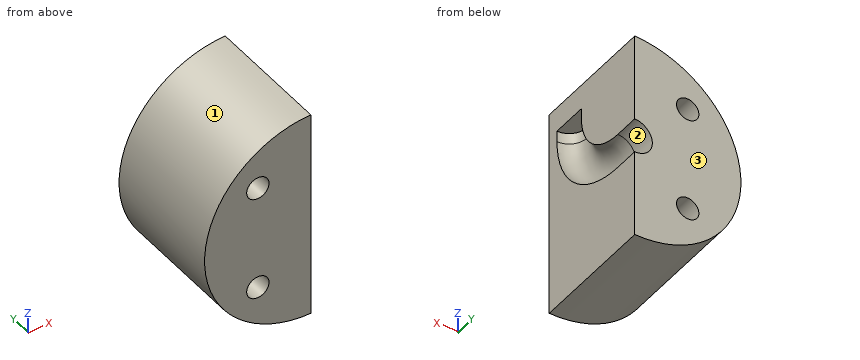
Autodesk Inventor part; units mm, degrees
ref_plane "YZ Plane" through (0, 0, 0) normal (1, 0, 0) x (0, 1, 0)
ref_plane "XZ Plane" through (0, 0, 0) normal (0, 1, 0) x (-1, 0, 0)
ref_plane "XY Plane" through (0, 0, 0) normal (0, 0, 1) x (1, 0, 0)
sketch "Sketch1" plane through (0, 0, 0) normal (0, 1, 0) x (-1, 0, 0)
  circle A0 centre (0, 0) radius 12.065
  line L0 (0, 0) -> (6.0168, -6.0168)
  line L1 (0, 0) -> (8.509, 0) construction
  circle A1 centre (6.0168, -6.0168) radius 1.27
  circle A2 centre (6.0168, 6.0168) radius 1.27
  circle A3 centre (-6.0168, 6.0168) radius 1.27
  circle A4 centre (-6.0168, -6.0168) radius 1.27
  dimension "d0" = 24.13
  dimension "d1" = 45
  dimension "d2" = 8.509
  dimension "d3" = 2.54
  dimension "d6" = 360
extrude "Extrusion1" add sketch "Sketch1" along normal blind 13.97
sketch "Sketch2" plane through (0, 0, 0) normal (1, 0, 0) x (0, 1, 0)
  line L0 (13.97, -12.065) -> (13.97, 12.065)
  line L1 (13.97, 0) -> (11.2075, 0)
  line L2 (11.2075, 0) -> (3.27, 0)
  line L3 (3.27, 0) -> (3.27, 7.9375)
  line L4 (3.27, 7.9375) -> (3.27, 9.2075)
  line L5 (0, 12.065) -> (0, -12.065)
  arc A0 (3.27, 7.9375) -> (11.2075, 0) centre (11.2075, 7.9375) ccw
  point P0 (0, 0)
  dimension "d15" = 7.9375
  dimension "d16" = 7.9375
  dimension "d17" = 1.27
  dimension "d18" = 3.27
sketch "Sketch3" plane through (0, 13.97, 0) normal (0, 1, 0) x (1, 0, 0)
  circle A0 centre (0, 0) radius 2
  dimension "d14" = 4
sweep "Sweep1" cut profiles "Sketch3" path "Sketch2" path curves L1 A0 L4
sketch "Sketch4" plane through (0, 0, 0) normal (1, 0, 0) x (0, 1, 0)
  line L0 (21.6749, -17.4359) -> (-6.3985, -17.4359)
  line L1 (-6.3985, -17.4359) -> (-6.3985, 17.036)
  line L2 (-6.3985, 17.036) -> (21.6749, 17.036)
  line L3 (21.6749, 17.036) -> (21.6749, -17.4359)
  point P0 (0, 0)
extrude "Extrusion2" cut sketch "Sketch4" along normal through all
properties part number "Side1Attachment" material "ABS Plastic"
CAD build for the part. Positions are in the model's coordinates, mm. Face numbers are marked on the shaded views. Round coordinates to 2 decimals unless told otherwise and drop trailing zeros. Order: outer loops, then holes, each group sorted by start corner. A loop starts at its lowest first (then second) coordinate and runs counter-clockwise, first axis right, second up. Notation, with made-up numbers: (-10, -3.5) - (-4, -3.5) arc R8 ccw to (-4, 5.5) - close; hole circle Ø7 at (46.5, -20.75). An arc over 180 degrees is marked (long way). Answer as CSV lines item,"result". Start each with the question number.
1. Drill centre lines: L1, parallel to Z at x = -6.75, y = 7.5; L2, parallel to Z at x = -6.5, y = 5; L3, parallel to Z at x = -1.75, y = 10.25. Where is each one in solid material? Low to high. Write a range as [from, to].
2. Saw through at D-D, the plane z = -9.25. Write the cut outline in (x, y).
3. Pull direction Z, two halves, no side cores. Call the marked faces 1, 2 and 3: +Z half, -Z half, draft (parallel to the pull), parting line (faces both ways), or undercut.
4. Saw through at C-C, the plane x = -0.75. Write the cut outline in (y, z).
5. Saw through at B-B, the plane y = 12.5. Write the cut outline in (x, z) (3 decimals).
6. Pin check, flat tips, straight feed: pin 1 (8 mm diameter, centred on y = 10.5, z = 3, fed in from +X); pin 2 (1.6 mm diameter, centred on x = -1, y = 4, fed in from -Z); pin 3 (2 mm diameter, centred on x = -6, y = 8.5, fed in from -Z); pin 4 (4 mm diameter, centred on x = -3.5, y = 8.5, fed in from +Z). Stop position of each tip, or through.
7. Saw through at A-A, the plane z = -6.75. Write the cut outline in (x, y).
Model answer:
1,L1,"z = [-10, -7.05], [-4.98, 4.98], [7.05, 10]"
1,L2,"z = [-10.16, -7.19], [-4.84, 4.84], [7.19, 10.16]"
1,L3,"z = [-11.94, -0.92], [1.03, 11.94]"
2,outline,"(-7.75, 0) - (0, 0) - (0, 13.97) - (-7.75, 13.97) - close"
3,face 1,"parting line"
3,face 2,"undercut"
3,face 3,"draft"
4,outline,"(0, -12.04) - (13.97, -12.04) - (13.97, -1.85) - (11.21, -1.85) arc R9.79 cw to (1.42, 7.94) - (1.42, 9.21) - (5.12, 9.21) - (5.12, 7.94) arc R6.08 ccw to (11.21, 1.85) - (13.97, 1.85) - (13.97, 12.04) - (0, 12.04) - close"
5,outline,"(0, -12.065) - (0, -2) arc R2 cw to (0, 2) - (0, 12.065) arc R12.065 ccw to start; hole circle Ø2.54 at (-6.017, -6.017); hole circle Ø2.54 at (-6.017, 6.017)"
6,pin 1,"stops at x = 0"
6,pin 2,"stops at z = -12.06"
6,pin 3,"stops at z = -10.98"
6,pin 4,"stops at z = 11.97"
7,outline,"(-10, 0) - (-7.05, 0) - (-7.05, 13.97) - (-10, 13.97) - close; (-4.98, 0) - (0, 0) - (0, 13.97) - (-4.98, 13.97) - close"
